Part model, mm, in its own coordinate system. A direction names the side the tool comes from. Round coordinates to 2 decimals unless told otherwise and drop trailing zeros. Loops run counter-clockwise (first coordinate to the right, second up) from the corner with the lowest first, then second, coordinate; pieces in that order, holes last. Notation, with made-up numbers: (33, 27) -> (79, 27) arc R33 ccw to (79, 56) -> close; hole circle Ø9 at (66, -4.75). An arc over 180 degrees is marked (long way). Answer as a JSON object with one key per item and string values. Group by question number.
from build123d import *

# Parameters (mm, degrees)
F1_DEPTH = 63.5
F0_W     = 25.1798671365
F0_H     = 19.05
F2_DEPTH = 25.4
F3_DEPTH = 7.9375
F5_R     = 5.08


with BuildPart() as f1:
    # F0 (on Front) → F1 (new body, symmetric)
    with BuildSketch(Plane.XZ):
        Polygon((41.275, -9.525), (41.275, 9.525), (22.225, 9.525), (-41.275, 9.525), (-41.275, -9.525), align=None)
    extrude(amount=F1_DEPTH, both=True)

    # F0 (on Front) → F2 (join, symmetric)
    with BuildSketch(Plane.XZ):
        with BuildLine():
            Line((22.225, 9.525), (41.275, 9.525))
            Line((41.275, 9.525), (41.275, 28.575))
            ThreePointArc((41.275, 28.575), (43.7066106583, 37.0183943417), (50.2565317176, 42.8752))
            Line((50.2565317176, 42.8752), (60.325, 42.8752))
            Line((60.325, 42.8752), (60.325, 61.9252))
            Line((60.325, 61.9252), (46.7808252517, 61.9252))
            ThreePointArc((46.7808252517, 61.9252), (29.0261751083, 49.2826338209), (22.225, 28.575))
            Line((22.225, 28.575), (22.225, 9.525))
        make_face()
        with Locations((72.9149335682, 52.4002)):
            Rectangle(F0_W, F0_H)
    extrude(amount=F2_DEPTH, both=True)

    # F0 (on Front) → F3 (join, symmetric)
    with BuildSketch(Plane.XZ):
        with BuildLine():
            Line((-41.275, 9.525), (22.225, 9.525))
            Line((22.225, 9.525), (22.225, 28.575))
            ThreePointArc((22.225, 28.575), (29.0261751083, 49.2826338209), (46.7808252517, 61.9252))
            add(Edge.make_bspline(
                [(-41.275, 9.525), (-40.1955842972, 39.3650457263), (14.7107355297, 61.2183064222), (46.7808252517, 61.9252)],
                knots=[0, 0, 0, 0, 102.4676013226, 102.4676013226, 102.4676013226, 102.4676013226], degree=3))
        make_face()
    extrude(amount=F3_DEPTH, both=True)

    # F0 (on Front) → F4 (revolve)
    with BuildSketch(Plane.XZ):
        Polygon((85.5048671365, 61.9252), (85.5048671365, 42.8752), (85.725, 42.8752), (85.725, 38.1), (111.125, 38.1), (111.125, 66.675), (85.5048671365, 66.675), align=None)
    revolve(axis=Axis((85.5048671365, 0, 52.5966957748), (0, 0, 1)))

    # F5
    f5_edges = [f1.edges().sort_by_distance(p)[0] for p in [
        (-41.275, -63.5, 0),
        (41.275, -63.5, 0),
        (41.275, 63.5, 0),
        (-41.275, 63.5, 0),
    ]]
    fillet(f5_edges, radius=F5_R)


solid = f1.part
Item 1: Band-saw the part on B-B, the plane x = 80. List the corners of the cut face in (y, z) (3 decimals), plus the area to 3 significant figures.
Item 2: Band-saw the part on C-C, the plane y = 46. List the corners of the cut face in (x, z) (3 decimals).
Item 3: Drop flat-ended pins along their axis: pin 1 Ø14 at (y, z) = (16, 22) entering from -X (3 decimals); pin 2 Ø3 at (y, z) = (-9.5, 14.5) entering from +X (3 decimals); pin 3 Ø9.5 at (x, y) = (62, 2.5) entering from -Z. Give the stop position or say it passes through.
Item 4: Two-plate mould, pull along X, no slides. Class faces 5 (the face through (43.64, -0.36, 36.91)), 6 (the face through (-41.275, -1, 0)), 7 (the face through (45, -25.4, 42)): pulls with the +X half, pulls with the -X half, needs draft (parallel to the pull), parting line crosses it, or undercut.
Item 5: Drill centre lines: line 1 (Y direction, x = 21, z = 44); line 2 (Z direction, x = 96.5, y = 16) (3 decimals); line 3 (Z direction, x = -14.5, y = 16) (3 decimals). Where is each one in solid material? Low to high.
Item 6: Which spindle directions (+Z, -Z, +X, -X, +Y, -Y) get a long thin tool onto all of the face, cutting with end or side? Do faces 1 (the face through (22.225, 17, 19)), 2 (the face through (22.225, -17, 19)), 3 (the face through (57, 0, 61.925)), 4 (the face through (41.275, -1, 5)). Say none if no direction does.
Item 7: Band-saw the part on A-A, the plane z = 7. List the corners of the cut face in (x, y) (3 decimals), plus the area to 3 significant figures.
Item 8: Band-saw the part on D-D, the plane y = 12.5. List the corners of the cut face in (x, z) (3 decimals).
Entries:
{
 "1": {"outline": "(-25.4, 42.875) -> (-25.022, 42.875) -> (-25.022, 38.1) -> (25.022, 38.1) -> (25.022, 42.875) -> (25.4, 42.875) -> (25.4, 61.925) -> (25.022, 61.925) -> (25.022, 66.675) -> (-25.022, 66.675) -> (-25.022, 61.925) -> (-25.4, 61.925) -> close", "area": "1,440 mm²"},
 "2": {"outline": "(-41.275, -9.525) -> (41.275, -9.525) -> (41.275, 9.525) -> (-41.275, 9.525) -> close"},
 "3": {"pin 1": "x = 22.225", "pin 2": "x = 41.275", "pin 3": "z = 38.1"},
 "4": {"face 5": "undercut", "face 6": "pulls with the -X half", "face 7": "needs draft"},
 "5": {"line 1": "-7.94 to 7.94", "line 2": "38.1 to 66.675", "line 3": "-9.525 to 9.525"},
 "6": {"face 1": "+Z, -X, +Y", "face 2": "+Z, -X, -Y", "face 3": "+Z, -X", "face 4": "-Z, +X, +Y, -Y"},
 "7": {"outline": "(-41.275, -58.42) arc R5.08 ccw to (-36.195, -63.5) -> (36.195, -63.5) arc R5.08 ccw to (41.275, -58.42) -> (41.275, 58.42) arc R5.08 ccw to (36.195, 63.5) -> (-36.195, 63.5) arc R5.08 ccw to (-41.275, 58.42) -> close", "area": "10,500 mm²"},
 "8": {"outline": "(-41.275, -9.525) -> (41.275, -9.525) -> (41.275, 28.575) arc R15.875 cw to (50.257, 42.875) -> (63.141, 42.875) -> (63.141, 38.1) -> (107.869, 38.1) -> (107.869, 66.675) -> (63.141, 66.675) -> (63.141, 61.925) -> (46.781, 61.925) arc R34.925 ccw to (22.225, 28.575) -> (22.225, 9.525) -> (-41.275, 9.525) -> close"}
}
